Here's how the part is built. I have some questions about the finished solid (model axes, mm). Face numbers are marked on the shaded views. A direction names the side the tool comes from. Give positions to 0.01 mm unless a question says otherwise; leave off trailing zeros. Loops run counter-clockwise (first coordinate to the right, second up) from the corner with the lowest first, then second, coordinate; pieces in that order, holes last. Notation, with made-up numbers: (88.25, -24) - (127.25, -24) arc R27 cw to (127.25, 9) - close; hole circle Ø9 at (21, 24.25). An arc over 180 degrees is marked (long way). Return JSON: item names as keys, results as strings. Group by question number.
(1) I need wall thicknesses on probe 1 along Z at (x, y) = (22, -1); probe 2 along Y at (x, z) = (24, 18.25); probe 3 along X at (y, z) = (23, 14). Which ranges of each line are inside material? Lowest first, please. Write a range as [from, to].
(2) If we section it at A-A (x = 0): Please give me the cut outline in (y, z).
(3) On a 3-axis mill with a long thin cutter (end or side, diameter ignored), from which of +Z, -Z, +X, -X, +Y, -Y can I reach the whole of each face in a straight line? I mean the marked faces 4, 5 and 6. Say none if no direction works.
(4) For P1, Ø12, axis at x = -30.5, y = -20, coming from the -Z side; P2, Ø2, axis at x = -37, z = 13.5, coming from the +Y side; P3, Ø1.5, axis at y = 19, z = 8.5, coming from the +X side; P4, Ø2, axis at x = 24.5, y = 10.5, coming from the +Z side, each with a flat end and sliding along its axis, tell me the tip position at first contact or that it passes through.
(5) If we mould it in two halves opening along X, with no side actions, what happens to the marked faces 1, 2 and 3? For each: released by +X, released by -X, zero draft, split by the parting line, or undercut.
```python
from build123d import *

# Parameters (mm, degrees)
SKETCH1_R           = 35.5
SKETCH1_R_2         = 32.5
BOSS_EXTRUDE1_DEPTH = 20
SKETCH2_R           = 35.5
BOSS_EXTRUDE2_DEPTH = 5
BOSS_EXTRUDE5_START = -10
BOSS_EXTRUDE5_DEPTH = 10
SKETCH6_R           = 2.1
CUT_EXTRUDE1_DEPTH  = 10
FILLET1_R           = 2
FILLET2_R           = 1


with BuildPart() as part:
    # Sketch1 → Boss-Extrude1 (new body)
    with BuildSketch(Plane.XY):
        Circle(SKETCH1_R)
        Circle(SKETCH1_R_2, mode=Mode.SUBTRACT)
    extrude(amount=BOSS_EXTRUDE1_DEPTH)

    # Sketch2 → Boss-Extrude2 (add)
    with BuildSketch(Plane(origin=(0, 0, 0), x_dir=(-1, 0, 0), z_dir=(0, 0, -1))):
        with Locations(Location((0, 0, 0), (0, 0, 180))):
            Circle(SKETCH2_R)
    extrude(amount=-BOSS_EXTRUDE2_DEPTH)

    # Sketch5 → Boss-Extrude5 (add)
    with BuildSketch(Plane.XY.offset(20).offset(BOSS_EXTRUDE5_START)):
        with BuildLine():
            Line((-44.01983555, 2.462594057), (-35.152395855, -4.955710406))
            ThreePointArc((-35.152395855, -4.955710406), (-35.21119146, 4.519070252), (-32.761689436, 13.671931294))
            Line((-32.761689436, 13.671931294), (-44.080202136, 10.462366296))
            ThreePointArc((-44.080202136, 10.462366296), (-48.049904962, 6.432296883), (-44.01983555, 2.462594057))
        make_face()
        with BuildLine():
            Line((44.080202136, 10.462366296), (32.761689436, 13.671931294))
            ThreePointArc((32.761689436, 13.671931294), (35.21119146, 4.519070252), (35.152395855, -4.955710406))
            Line((35.152395855, -4.955710406), (44.01983555, 2.462594057))
            ThreePointArc((44.01983555, 2.462594057), (48.049904962, 6.432296883), (44.080202136, 10.462366296))
        make_face()
    extrude(amount=BOSS_EXTRUDE5_DEPTH)

    # Sketch6 → Cut-Extrude1 (cut)
    with BuildSketch(Plane(origin=(0, 0, 10), x_dir=(-1, 0, 0), z_dir=(0, 0, -1))):
        with Locations((-44.050018843, 6.462480176)):
            Circle(SKETCH6_R)
        with Locations((44.050018843, 6.462480176)):
            Circle(SKETCH6_R)
    extrude(amount=-CUT_EXTRUDE1_DEPTH, mode=Mode.SUBTRACT)

    # Fillet1
    fillet1_edges = [part.edges().sort_by_distance(p)[0] for p in [
        (-35.21119146, 4.519070252, 10),
        (-32.761689436, 13.671931294, 15),
        (-35.152395855, -4.955710406, 15),
        (34.808691264, 6.971729521, 10),
        (35.152395855, -4.955710406, 15),
        (32.761689436, 13.671931294, 15),
    ]]
    fillet(fillet1_edges, radius=FILLET1_R)

    # Fillet2
    fillet2_edges = [part.edges().sort_by_distance(p)[0] for p in [
        (-32.5, 0, 5),
        (-35.5, 0, 0),
        (-39.876382255, -1.003727579, 20),
        (38.877374536, 11.937720328, 20),
        (0, -35.5, 20),
        (0, 35.5, 20),
        (-32.5, 0, 20),
        (-38.877374536, 11.937720328, 20),
        (39.876382255, -1.003727579, 20),
        (-35.278088778, -5.014669945, 20),
        (-32.912138626, 13.824247135, 20),
        (32.912138626, 13.824247135, 20),
        (35.278088778, -5.014669945, 20),
    ]]
    fillet(fillet2_edges, radius=FILLET2_R)


solid = part.part
```
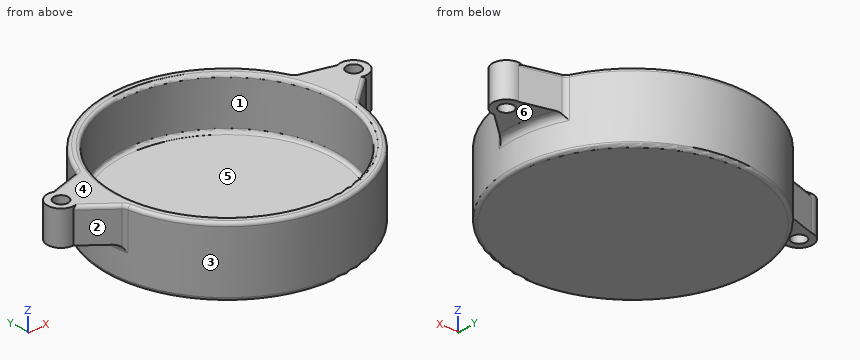
Values:
{
 "1": {"probe 1": "[0, 5]", "probe 2": "[-26.16, -21.91], [21.91, 26.16]", "probe 3": "[-27.04, -22.96], [22.96, 27.04]"},
 "2": {"outline": "(-35.5, 1) arc R1 ccw to (-34.5, 0) - (34.5, 0) arc R1 ccw to (35.5, 1) - (35.5, 19) arc R1 ccw to (34.5, 20) - (33.5, 20) arc R1 ccw to (32.5, 19) - (32.5, 6) arc R1 cw to (31.5, 5) - (-31.5, 5) arc R1 cw to (-32.5, 6) - (-32.5, 19) arc R1 ccw to (-33.5, 20) - (-34.5, 20) arc R1 ccw to (-35.5, 19) - close"},
 "3": {"face 4": "+Z, +X, -X, +Y, -Y", "face 5": "+Z", "face 6": "-Z, +X, +Y"},
 "4": {"P1": "z = 0", "P2": "y = 12.75", "P3": "x = 30.45", "P4": "z = 5"},
 "5": {"face 1": "undercut", "face 2": "released by -X", "face 3": "split by the parting line"}
}
